The model under review builds one solid part; all positions refer to its coordinate system, in mm. A direction names the side the tool comes from. Coordinates: 2 decimals unless noted, no trailing zeros. Write each loop counter-clockwise with the first axis right and the second up, starting at its lowest first coordinate (ties: lowest second). Pieces come first, ordered by that corner, then holes.
1) Add section A-A, the plane x = -22.86. State the section outline as (y, z) points (3 decimals).
2) Machinability: for faces 1 (the flat face through (-12.7, 3, 43)), 2 (the flat face through (8, 6.35, -1)), 3 (the flat face through (-12.7, 3, -42)), which of the approach directions +Z, -Z, +X, -X, +Y, -Y give a long, thin tool a straight path to every point of the face, cutting with its end or side? Answer none if there is none.
3) Add section C-C, the plane y = 4.25. State the section outline as (x, z) points (3 decimals), then the cut area to 3 significant figures.
4) Add section B-B, the plane z = 0. State the section outline as (x, y) points (3 decimals).
5) For line 1 (X direction, y = 2.25, z = 0) (3 decimals); line 2 (X direction, y = 5.25, z = 39); line 3 (Z direction, x = -31.5, y = 4), list the stretches that pass through material, from the lowest coordinate up.
6) For P1, Ø1.9, axis at y = 4, z = -40, coming from the -X side, flat-tipped, find the tip position at first contact; note if it passes through.
7) Mouldability with a two-part tool opening along Z and no side actions: class faces 4 (the flat face through (12, 3, 57.15)), 5 (the cylindrical face through (-35.817, 3.131, 6.739)), 6 (the flat face through (8, 0, -1)), 7 (the flat face through (-22, 3, -27.94)) as released by +Z, released by -Z, zero draft, split by the parting line, or undercut.
from build123d import *

# Parameters (mm, degrees)
SKETCH1_W           = 76.2
SKETCH1_H           = 114.3
SKETCH1_R           = 14.605
BOSS_EXTRUDE1_DEPTH = 6.35
CUT_EXTRUDE1_REACH  = 70.979
SKETCH2_W           = 25.4
SKETCH2_H           = 29.21
CUT_EXTRUDE3_REACH  = 70.979


with BuildPart() as part:
    # Sketch1 → Boss-Extrude1 (new body)
    with BuildSketch(Plane(origin=(0, 0, 0), x_dir=(1, 0, 0), z_dir=(0, 1, 0))):
        Rectangle(SKETCH1_W, SKETCH1_H)
        with Locations(Location((-22.86, 0, 0), (0, 0, 270))):
            Circle(SKETCH1_R, mode=Mode.SUBTRACT)
    extrude(amount=BOSS_EXTRUDE1_DEPTH)

    # Sketch2 → Cut-Extrude1 (cut, up to next)
    with BuildSketch(Plane(origin=(0, 6.35, 0), x_dir=(1, 0, 0), z_dir=(0, 1, 0)), mode=Mode.PRIVATE) as cut_extrude1_sk1:
        with Locations((-25.4, 42.545)):
            Rectangle(SKETCH2_W, SKETCH2_H)
    cut_extrude1_tool1 = extrude(cut_extrude1_sk1.sketch, amount=-CUT_EXTRUDE1_REACH, mode=Mode.PRIVATE) & part.part
    # Sketch2 → Cut-Extrude1 (cut, up to next)
    with BuildSketch(Plane(origin=(0, 6.35, 0), x_dir=(1, 0, 0), z_dir=(0, 1, 0)), mode=Mode.PRIVATE) as cut_extrude1_sk2:
        with Locations((-25.4, -42.545)):
            Rectangle(SKETCH2_W, SKETCH2_H)
    cut_extrude1_tool2 = extrude(cut_extrude1_sk2.sketch, amount=-CUT_EXTRUDE1_REACH, mode=Mode.PRIVATE) & part.part
    add(cut_extrude1_tool1.solids().sort_by_distance((-25.4, 6.35, -42.545))[0], mode=Mode.SUBTRACT)
    add(cut_extrude1_tool2.solids().sort_by_distance((-25.4, 6.35, 42.545))[0], mode=Mode.SUBTRACT)

    # Sketch4 → Cut-Extrude3 (cut, up to next)
    with BuildSketch(Plane(origin=(0, 6.35, 0), x_dir=(1, 0, 0), z_dir=(0, 1, 0)), mode=Mode.PRIVATE) as cut_extrude3_sk1:
        Polygon((-31.75, -27.94), (-38.1, -15.24), (-38.1, -27.94), align=None)
    cut_extrude3_tool1 = extrude(cut_extrude3_sk1.sketch, amount=-CUT_EXTRUDE3_REACH, mode=Mode.PRIVATE) & part.part
    # Sketch4 → Cut-Extrude3 (cut, up to next)
    with BuildSketch(Plane(origin=(0, 6.35, 0), x_dir=(1, 0, 0), z_dir=(0, 1, 0)), mode=Mode.PRIVATE) as cut_extrude3_sk2:
        Polygon((-31.75, 27.94), (-38.1, 27.94), (-38.1, 15.24), align=None)
    cut_extrude3_tool2 = extrude(cut_extrude3_sk2.sketch, amount=-CUT_EXTRUDE3_REACH, mode=Mode.PRIVATE) & part.part
    add(cut_extrude3_tool1.solids().sort_by_distance((-35.983333, 6.35, 23.706667))[0], mode=Mode.SUBTRACT)
    add(cut_extrude3_tool2.solids().sort_by_distance((-35.983333, 6.35, -23.706667))[0], mode=Mode.SUBTRACT)


solid = part.part
Geometry results:
1. outline: (0, -27.94) - (6.35, -27.94) - (6.35, -14.605) - (0, -14.605) - close; (0, 14.605) - (6.35, 14.605) - (6.35, 27.94) - (0, 27.94) - close
2. face 1: +Z, -X, +Y, -Y
2. face 2: +Z, -Z, +X, -X, +Y
2. face 3: -Z, -X, +Y, -Y
3. outline: (-38.1, -15.24) - (-31.75, -27.94) - (-12.7, -27.94) - (-12.7, -57.15) - (38.1, -57.15) - (38.1, 57.15) - (-12.7, 57.15) - (-12.7, 27.94) - (-31.75, 27.94) - (-38.1, 15.24) - close; hole circle Ø29.21 at (-22.86, 0)
3. area: 6,480 mm2
4. outline: (-38.1, 0) - (-37.465, 0) - (-37.465, 6.35) - (-38.1, 6.35) - close; (-8.255, 0) - (38.1, 0) - (38.1, 6.35) - (-8.255, 6.35) - close
5. line 1: x = -38.1 to -37.465, -8.255 to 38.1
5. line 2: x = -12.7 to 38.1
5. line 3: z = -27.94 to -11.78, 11.78 to 27.94
6. P1: stops at x = -12.7
7. face 4: released by +Z
7. face 5: undercut
7. face 6: zero draft
7. face 7: released by -Z
